from build123d import *

# Parameters (mm, degrees)
SKETCH1_W           = 31.75
SKETCH1_H           = 6.35
SKETCH1_W_2         = 6.35
SKETCH1_H_2         = 50.8
SKETCH1_W_3         = 22.86
BOSS_EXTRUDE1_DEPTH = 6.35
FILLET1_R           = 2.54
FILLET2_R           = 1.27


with BuildPart() as part:
    # Sketch1 → Boss-Extrude1 (new body)
    with BuildSketch(Plane.XY):
        with Locations((22.225, 47.625)):
            Rectangle(SKETCH1_W, SKETCH1_H)
        with Locations((3.175, 25.4)):
            Rectangle(SKETCH1_W_2, SKETCH1_H_2)
        with Locations((17.78, 25.4)):
            Rectangle(SKETCH1_W_3, SKETCH1_H)
        with Locations((22.225, 3.175)):
            Rectangle(SKETCH1_W, SKETCH1_H)
    extrude(amount=BOSS_EXTRUDE1_DEPTH)

    # Fillet1
    fillet1_edges = [part.edges().sort_by_distance(p)[0] for p in [
        (6.35, 44.45, 3.175),
        (6.35, 28.575, 3.175),
        (6.35, 22.225, 3.175),
        (6.35, 6.35, 3.175),
    ]]
    fillet(fillet1_edges, radius=FILLET1_R)

    # Fillet2
    fillet2_edges = [part.edges().sort_by_distance(p)[0] for p in [
        (0, 0, 3.175),
        (0, 50.8, 3.175),
    ]]
    fillet(fillet2_edges, radius=FILLET2_R)


solid = part.part
Source: CAD feature listing. Evaluate the final solid. Frame: model axes, mm. A direction names the side the tool comes from. Coordinates: 2 decimals unless noted, no trailing zeros. Write each loop counter-clockwise with the first axis right and the second up, starting at its lowest first coordinate (ties: lowest second). Pieces come first, ordered by that corner, then holes. Notation, with made-up numbers: M 83,10 L 129,10 A29 ccw 129,36 Z; hole C 82,40.25 d11. An arc over 180 degrees is marked long. Use a Markdown table: item, result.
1) First-contact query: pin 1 Ø3 at (y, z) = (26, 4.5) entering from +X; pin 2 Ø3 at (x, y) = (20, 30.5) entering from -Z; pin 3 Ø3 at (y, z) = (15, 3.5) entering from +X. Flat tips, straight axial feed; report the tip coordinate or a pass-through.
Conclusion:
| item | result |
|---|---|
| pin 1 | stops at x = 29.21 |
| pin 2 | passes through |
| pin 3 | stops at x = 6.35 |
2) Ray query, L1, parallel to Y at x = 23, z = 4.75 (3 decimals); L2, parallel to Y at x = 33, z = 0.75. Return the intervals inside material, ascending.
Conclusion:
| item | result |
|---|---|
| L1 | y = 0 to 6.35, 22.225 to 28.575, 44.45 to 50.8 |
| L2 | y = 0 to 6.35, 44.45 to 50.8 |
3) Section B-B, the plane z = 3. Output: boundary loops of the cut face in (x, y) (3 decimals), then the cut area to 3 significant figures.
Conclusion:
| item | result |
|---|---|
| outline | M 0,1.27 A1.27 ccw 1.27,0 L 38.1,0 L 38.1,6.35 L 8.89,6.35 A2.54 cw 6.35,8.89 L 6.35,19.685 A2.54 cw 8.89,22.225 L 29.21,22.225 L 29.21,28.575 L 8.89,28.575 A2.54 cw 6.35,31.115 L 6.35,41.91 A2.54 cw 8.89,44.45 L 38.1,44.45 L 38.1,50.8 L 1.27,50.8 A1.27 ccw 0,49.53 Z |
| area | 876 mm^2 |
4) Mould query, pull axis Y, two halves, no side actions, for faces 3 (the cylindrical face through (7.114, 29.299, 3.219)), 4 (the cylindrical face through (0.362, 0.382, 3.219)), 5 (the flat face through (15, 26, 0)). Classes: pulls with the +Y half, pulls with the -Y half, needs draft (parallel to the pull), parting line crosses it, or undercut.
Conclusion:
| item | result |
|---|---|
| face 3 | undercut |
| face 4 | pulls with the -Y half |
| face 5 | needs draft |
5) Section C-C, the plane x = 32. Output: boundary loops of the cut face in (y, z).
Conclusion:
| item | result |
|---|---|
| outline | M 0,0 L 6.35,0 L 6.35,6.35 L 0,6.35 Z; M 44.45,0 L 50.8,0 L 50.8,6.35 L 44.45,6.35 Z |
6) Reachability of faces 1 (the cylindrical face through (0.382, 50.438, 3.219)), 2 (the flat face through (23, 6.35, 3)) from +Z, -Z, +X, -X, +Y, -Y: full face, straight path, thin tool, end or side. Return the list, or none.
Conclusion:
| item | result |
|---|---|
| face 1 | +Z, -Z, -X, +Y |
| face 2 | +Z, -Z, +X |
7) Section D-D, the plane y = 24.5. Output: boundary loops of the cut face in (x, z).
Conclusion:
| item | result |
|---|---|
| outline | M 0,0 L 29.21,0 L 29.21,6.35 L 0,6.35 Z |
8) Section A-A, the plane x = 10.5. Output: boundary loops of the cut face in (y, z) (3 decimals).
Conclusion:
| item | result |
|---|---|
| outline | M 0,0 L 6.35,0 L 6.35,6.35 L 0,6.35 Z; M 22.225,0 L 28.575,0 L 28.575,6.35 L 22.225,6.35 Z; M 44.45,0 L 50.8,0 L 50.8,6.35 L 44.45,6.35 Z |
